```python
from build123d import *

# Parameters (mm, degrees)
SKETCH_W     = 145
SKETCH_H     = 60
PAD_DEPTH    = 21
THICKNESS_T  = -2
SKETCH001_W  = 130
SKETCH001_H  = 19
POCKET_DEPTH = 2
SKETCH002_R  = 1.5
PAD001_DEPTH = 4


with BuildPart() as part:
    # Sketch → Pad (new body)
    with BuildSketch(Plane.XY):
        Rectangle(SKETCH_W, SKETCH_H)
    extrude(amount=PAD_DEPTH)

    # Thickness
    thickness_openings = [part.faces().sort_by_distance(p)[0] for p in [
        (0, 0, 21),
    ]]
    offset(amount=THICKNESS_T, openings=thickness_openings)

    # Sketch001 (on Face3 of Thickness) → Pocket (cut)
    with BuildSketch(Plane.XZ.offset(30)):
        with Locations((0, 11.5)):
            Rectangle(SKETCH001_W, SKETCH001_H)
    extrude(amount=-POCKET_DEPTH, mode=Mode.SUBTRACT)

    # Sketch002 (on Face15 of Pocket) → Pad001 (join)
    with BuildSketch(Plane.XY.offset(2)):
        with Locations((-67, 18.5)):
            Circle(SKETCH002_R)
        with Locations((-67, -21.5)):
            Circle(SKETCH002_R)
        with Locations((65.5, 18.5)):
            Circle(SKETCH002_R)
        with Locations((65.5, -21.5)):
            Circle(SKETCH002_R)
    extrude(amount=PAD001_DEPTH)


solid = part.part
```
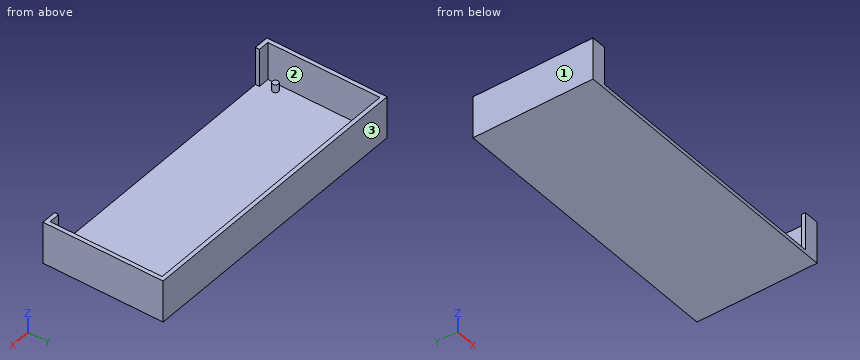
CAD build for the part. Positions are in the model's coordinates, mm. Face numbers are marked on the shaded views. Give positions to 0.01 mm unless a question says otherwise; leave off trailing zeros. Order: outer loops, then holes, each group sorted by start corner. A loop starts at its lowest first (then second) coordinate and runs counter-clockwise, first axis right, second up. Notation, with made-up numbers: M 39.25,7 L 86.25,7 A28 ccw 86.25,28 Z; hole C 18,-18 d5. An arc over 180 degrees is marked long. Put each result on its own line as item: value. Start each with the question number.
(1) Drill centre lines: line 1 along X through (y, z) = (1, 4); line 2 along Y through (x, z) = (33.5, 7); line 3 along Z through (x, y) = (2.5, -11.5). Where is each one in solid material? Low to high.
(2) Saw through at C-C, the plane x = -4.5. Write the cut outline in (y, z), then the cut area to 3 significant figures.
(3) Saw through at A-A, the plane y = 21.5. Write the cut outline in (x, z).
(4) Saw through at B-B, the plane z = 9.25. Write the cut outline in (x, y).
(5) Mould opens along Y. For the marked faces 1, 2 and 3 say: +Y half, -Y half, draft (parallel to the pull), parting line (faces both ways), or undercut.
(6) Flat gauge pins, fed straight in: pin 1 Ø1.5 at (x, y) = (65, -21.5) entering from +Z; pin 2 Ø4 at (x, y) = (38.5, -14.5) entering from -Z; pin 3 Ø2 at (x, z) = (-29.5, 6) entering from -Y; pin 4 Ø6 at (x, y) = (-10, 18.5) entering from +Z. Where does each tip first touch, or does it go through?
(7) Saw through at D-D, the plane y = -21.5. Write the cut outline in (x, z).
Check result:
1. line 1: x = -72.5 to -70.5, 70.5 to 72.5
1. line 2: y = 28 to 30
1. line 3: z = 0 to 2
2. outline: M -30,0 L 30,0 L 30,21 L 28,21 L 28,2 L -30,2 Z
2. area: 158 mm2
3. outline: M -72.5,0 L 72.5,0 L 72.5,21 L 70.5,21 L 70.5,2 L -70.5,2 L -70.5,21 L -72.5,21 Z
4. outline: M -72.5,-30 L -65,-30 L -65,-28 L -70.5,-28 L -70.5,28 L 70.5,28 L 70.5,-28 L 65,-28 L 65,-30 L 72.5,-30 L 72.5,30 L -72.5,30 Z
5. face 1: draft
5. face 2: undercut
5. face 3: +Y half
6. pin 1: stops at z = 6
6. pin 2: stops at z = 0
6. pin 3: stops at y = 28
6. pin 4: stops at z = 2
7. outline: M -72.5,0 L 72.5,0 L 72.5,21 L 70.5,21 L 70.5,2 L 67,2 L 67,6 L 64,6 L 64,2 L -65.5,2 L -65.5,6 L -68.5,6 L -68.5,2 L -70.5,2 L -70.5,21 L -72.5,21 Z
